The model under review builds one solid part; all positions refer to its coordinate system, in mm. Face numbers are marked on the shaded views. A direction names the side the tool comes from. Coordinates: 2 decimals unless noted, no trailing zeros. Order: outer loops, then holes, each group sorted by start corner. A loop starts at its lowest first (then second) coordinate and runs counter-clockwise, first axis right, second up. Notation, with made-up numbers: (66.25, 27.5) -> (88.25, 27.5) arc R7 ccw to (88.25, 40.5) -> close; hole circle Ø11 at (78, -6). An arc over 180 degrees is marked (long way). Use one line per item in the form item = value.
from build123d import *

# Parameters (mm, degrees)
BOSS_EXTRUDE1_DEPTH = 100
FILLET1_R           = 1


with BuildPart() as part:
    # Sketch1 → Boss-Extrude1 (new body)
    with BuildSketch(Plane(origin=(0, 0, 0), x_dir=(1, 0, 0), z_dir=(0, 1, 0))):
        Polygon((0, 0), (20, 0), (20, -2), (7, -2), (7, -9), (0, -9), (0, -7), (5, -7), (5, -2), (0, -2), align=None)
    extrude(amount=BOSS_EXTRUDE1_DEPTH)

    # Fillet1
    fillet1_edges = [part.edges().sort_by_distance(p)[0] for p in [
        (20, 50, 2),
        (7, 50, 2),
        (7, 50, 9),
        (0, 50, 7),
        (0, 50, 2),
    ]]
    fillet(fillet1_edges, radius=FILLET1_R)


solid = part.part
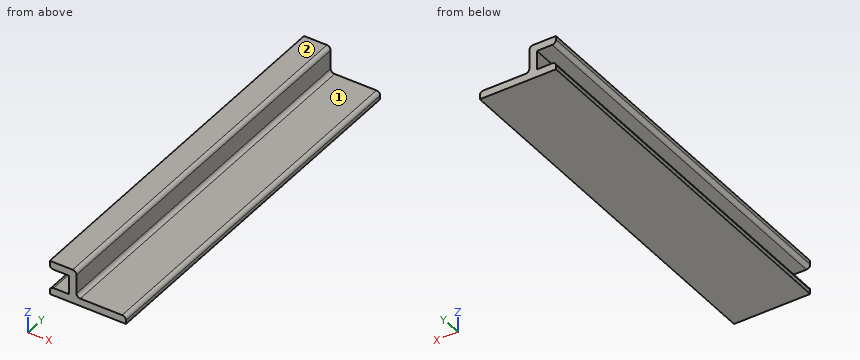
Item 1: Tool access review of the marked faces 1 and 2: name each direction out of +Z, -Z, +X, -X, +Y, -Y from which nothing blocks a thin tool from reaching the whole face with its end or side.
Results found:
face_1 = +Z, +X, +Y, -Y
face_2 = +Z, +X, -X, +Y, -Y
Item 2: To check wall thickness, follow L1, parallel to Z at x = 4.5, y = 71.5; L2, parallel to X at y = 83, z = 4.75; L3, parallel to Z at x = 13.5, y = 80. State the ranges of each line that lie inside material, in increasing order. Write a range as from..to.
Results found:
L1 = 0..2, 7..9
L2 = 5..7
L3 = 0..2
Item 3: Clearance check with flat-ended pins moving along their axes: pin 1 (5.5 mm diameter, centred on x = 11, y = 42, fed in from +Z); pin 2 (2.5 mm diameter, centred on y = 65, z = 5, fed in from -X); pin 3 (1 mm diameter, centred on y = 51, z = 4.5, fed in from +X). State where each tip first meets the part, or that it passes through.
Results found:
pin_1 = 2
pin_2 = 5
pin_3 = 7
Item 4: We need section A-A (y = 24.5). Write out the cut boundary in (x, z).
Results found:
outline = (0, 0) -> (20, 0) -> (20, 1) arc R1 ccw to (19, 2) -> (8, 2) arc R1 cw to (7, 3) -> (7, 8) arc R1 ccw to (6, 9) -> (0, 9) -> (0, 8) arc R1 ccw to (1, 7) -> (5, 7) -> (5, 2) -> (1, 2) arc R1 ccw to (0, 1) -> close
Item 5: We need section B-B (x = 15.25). Write out the cut boundary in (y, z).
Results found:
outline = (0, 0) -> (100, 0) -> (100, 2) -> (0, 2) -> close
